Source: CAD feature listing. Evaluate the final solid. Frame: model axes, mm. Face numbers are marked on the shaded views. Coordinates: 2 decimals unless noted, no trailing zeros. Write each loop counter-clockwise with the first axis right and the second up, starting at its lowest first coordinate (ties: lowest second). Pieces come first, ordered by that corner, then holes. Notation, with made-up numbers: M -21,6 L -3,6 A37 ccw -3,43 Z; hole C 17.5,56 d8. An arc over 180 degrees is marked long. Answer as CSV lines item,"result". Start each with the question number.
1. Section A-A on y = 6. Return the cut outline in (x, z).
2. Contact query for flat-ended pins moving along their axis: pin 1 Ø1.5 at (x, y) = (-3, 4) entering from +Z; pin 2 Ø1 at (x, z) = (1.5, 3) entering from -Y; pin 3 Ø3 at (y, z) = (3, 0.5) entering from +X. Output: stop coordinate, or through.
3. Mould query, pull axis Z, two halves, no side actions, for the marked faces 1, 2 and 3. Classes: pulls with the +Z half, pulls with the -Z half, needs draft (parallel to the pull), parting line crosses it, or undercut.
4. Line query: probe 1 along Z at (x, y) = (0, 12.4); probe 2 along Y at (x, z) = (-2.75, 0.5). Output: solid intervals per line, ascending. Write a range as [from, to].
```python
from build123d import *

# Parameters (mm, degrees)
CROQUIS1_R            = 4.1
EXTRUIR1_DEPTH        = 12.5
CROQUIS2_R            = 1.721107575
REDONDEO1_R           = 0.5
REDONDEO2_R           = 1.5
CROQUIS3_R            = 3.23696878
CORTAR_EXTRUIR1_DEPTH = 0.2


with BuildPart() as part:
    # Croquis1 → Extruir1 (new body)
    with BuildSketch(Plane(origin=(0, 0, 0), x_dir=(1, 0, 0), z_dir=(0, 1, 0))):
        Circle(CROQUIS1_R)
    extrude(amount=EXTRUIR1_DEPTH)

    # Croquis2 → Cortar-Revolución1 (revolve, cut)
    with BuildSketch(Plane(origin=(0, 0, 0), x_dir=(0, 0, -1), z_dir=(1, 0, 0))):
        with Locations((5.382002142, 2.987795872)):
            Circle(CROQUIS2_R)
    revolve(axis=Axis((0, 12.5, 0), (0, 1, 0)), mode=Mode.SUBTRACT)

    # Redondeo1
    redondeo1_edges = [part.edges().sort_by_distance(p)[0] for p in [
        (-4.1, 0, 0),
        (-4.1, 12.5, 0),
    ]]
    fillet(redondeo1_edges, radius=REDONDEO1_R)

    # Redondeo2
    redondeo2_edges = [part.edges().sort_by_distance(p)[0] for p in [
        (2.899137803, 4.136134582, -2.899137803),
        (-2.899137803, 1.839457161, 2.899137803),
    ]]
    fillet(redondeo2_edges, radius=REDONDEO2_R)

    # Croquis3 → Cortar-Extruir1 (cut)
    with BuildSketch(Plane(origin=(0, 12.5, 0), x_dir=(1, 0, 0), z_dir=(0, 1, 0))):
        Circle(CROQUIS3_R)
    extrude(amount=-CORTAR_EXTRUIR1_DEPTH, mode=Mode.SUBTRACT)


solid = part.part
```
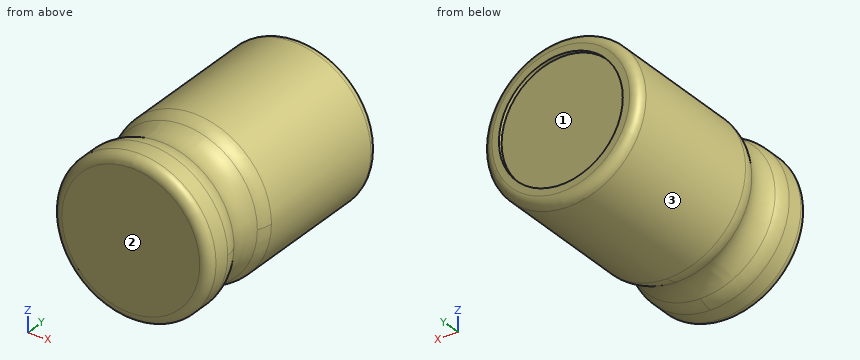
Values:
1,outline,"C 0,0 d8.2"
2,pin 1,"z = 3.35"
2,pin 2,"y = 0"
2,pin 3,"x = 4.09"
3,face 1,"undercut"
3,face 2,"needs draft"
3,face 3,"parting line crosses it"
4,probe 1,"[-3.9, -3.24], [3.24, 3.9]"
4,probe 2,"[0, 12.3]"
